The model under review builds one solid part; all positions refer to its coordinate system, in mm. A direction names the side the tool comes from. Give positions to 0.01 mm unless a question says otherwise; leave off trailing zeros. Loops run counter-clockwise (first coordinate to the right, second up) from the corner with the lowest first, then second, coordinate; pieces in that order, holes last. Notation, with made-up numbers: M 89,75.5 L 130,75.5 A35 cw 130,111.5 Z; hole C 37.5,45 d1. An arc over 180 degrees is marked long. Put each result on its own line as item: value. Start each with the question number.
from build123d import *

# Parameters (mm, degrees)
BOSS_EXTRUDE1_DEPTH     = 24
SKETCH2_R               = 2.05
SKETCH2_R_2             = 4
CUT_EXTRUDE1_DEPTH      = 45
CUT_EXTRUDE2_DEPTH      = 44.9089968
CUT_EXTRUDE2_DEPTH_BACK = 44.9089968
SKETCH3_R               = 4
SKETCH3_R_2             = 2
FILLET1_R               = 2


with BuildPart() as part:
    # Sketch1 → Boss-Extrude1 (new body)
    with BuildSketch(Plane.XY):
        Polygon((0, 0), (0, 26), (0, 28), (26, 28), (26, 26), (2, 26), (2, 2), (26, 2), (26, 0), align=None)
    extrude(amount=BOSS_EXTRUDE1_DEPTH)

    # Sketch2 → Cut-Extrude1 (cut, through all)
    with BuildSketch(Plane(origin=(2, 0, 0), x_dir=(0, 0, -1), z_dir=(1, 0, 0))):
        with Locations(Location((-12, 22, 0), (0, 0, 90))):
            Circle(SKETCH2_R)
        with Locations(Location((-12, 14, 0), (0, 0, 90))):
            Circle(SKETCH2_R_2)
        with Locations(Location((-6.343145751, 19.656854249, 0), (0, 0, 90))):
            Circle(SKETCH2_R)
        with Locations(Location((-4, 14, 0), (0, 0, 90))):
            Circle(SKETCH2_R)
        with Locations(Location((-6.343145751, 8.343145751, 0), (0, 0, 90))):
            Circle(SKETCH2_R)
        with Locations(Location((-12, 6, 0), (0, 0, 90))):
            Circle(SKETCH2_R)
        with Locations(Location((-17.656854249, 8.343145751, 0), (0, 0, 90))):
            Circle(SKETCH2_R)
        with Locations(Location((-20, 14, 0), (0, 0, 90))):
            Circle(SKETCH2_R)
        with Locations(Location((-17.656854249, 19.656854249, 0), (0, 0, 90))):
            Circle(SKETCH2_R)
    extrude(amount=-CUT_EXTRUDE1_DEPTH, mode=Mode.SUBTRACT)

    # Sketch3 → Cut-Extrude2 (cut, two sides: drawn at the far end of the back side and taken through both)
    with BuildSketch(Plane(origin=(0, 2, 0), x_dir=(1, 0, 0), z_dir=(0, 1, 0)).offset(-CUT_EXTRUDE2_DEPTH_BACK)):
        with Locations(Location((14, -12, 0), (0, 0, 270))):
            Circle(SKETCH3_R)
        with Locations(Location((22, -12, 0), (0, 0, 270))):
            Circle(SKETCH3_R_2)
        with Locations(Location((19.656854249, -17.656854249, 0), (0, 0, 270))):
            Circle(SKETCH3_R_2)
        with Locations(Location((14, -20, 0), (0, 0, 270))):
            Circle(SKETCH3_R_2)
        with Locations(Location((8.343145751, -17.656854249, 0), (0, 0, 270))):
            Circle(SKETCH3_R_2)
        with Locations(Location((6, -12, 0), (0, 0, 270))):
            Circle(SKETCH3_R_2)
        with Locations(Location((8.343145751, -6.343145751, 0), (0, 0, 270))):
            Circle(SKETCH3_R_2)
        with Locations(Location((14, -4, 0), (0, 0, 270))):
            Circle(SKETCH3_R_2)
        with Locations(Location((19.656854249, -6.343145751, 0), (0, 0, 270))):
            Circle(SKETCH3_R_2)
    extrude(amount=CUT_EXTRUDE2_DEPTH + CUT_EXTRUDE2_DEPTH_BACK, mode=Mode.SUBTRACT)

    # Fillet1
    fillet1_edges = [part.edges().sort_by_distance(p)[0] for p in [
        (26, 1, 0),
        (0, 0, 12),
        (0, 28, 12),
        (26, 27, 24),
        (26, 1, 24),
        (26, 27, 0),
    ]]
    fillet(fillet1_edges, radius=FILLET1_R)


solid = part.part
(1) Draft analysis for pull direction Y (two halves, no side actions). For faces 1 (the flat face through (17, 26, 9)), 2 (the cylindrical face through (1.014, 9.445, 19.385)), 3 (the cylindrical face through (0.57, 27.4, 12.17)), 4 (the cylindrical face through (20.8, 27, 10.4)), state which applies: +Y half, -Y half, draft (parallel to the pull), parting line (faces both ways), or undercut.
(2) We need section B-B, the plane z = 15. Write out the cut boundary in (x, y), plus the area to 3 significant figures.
(3) We need section D-D, the plane x = 23. Write out the cut boundary in (y, z), plus the area to 3 significant figures.
(4) For faces 5 (the flat face through (11, 2, 9)), 6 (the cylindrical face through (17.704, 26.986, 5.91)), list the 3-axis set-ups (+Z, -Z, +X, -X, +Y, -Y) from which the entire face can be reached by the end or side of a thin tool; tool diameter is ignored.
(5) To check wall thickness, follow L1, parallel to Z at x = 14, y = 27.55; L2, parallel to Y at x = 20.75, z = 14; L3, parallel to X at y = 26.9, z = 12. State the ranges of each line that lie inside material, in increasing order. Write a range as [from, to].
(6) We need section C-C, the plane y = 22.5. Write out the cut boundary in (x, z).
(7) Insertion check: pin 1 (6.5 mm diameter, centred on y = 19.66, z = 6.34, fed in from +X). The pin has a flat end and moves straight along its axis. Give the tip position at first contact, or say it passes through.
(8) We need section A-A, the plane x = 3. Write out the cut boundary in (y, z), plus the area to 3 significant figures.
Check sheet entries:
1. face 1: undercut
1. face 2: undercut
1. face 3: +Y half
1. face 4: draft
2. outline: M 0,2 A2 ccw 2,0 L 11.35,0 L 11.35,2 L 2,2 L 2,11.35 L 0,11.35 Z; M 0,16.65 L 2,16.65 L 2,26 L 11.35,26 L 11.35,28 L 2,28 A2 ccw 0,26 Z; M 16.65,0 L 26,0 L 26,2 L 16.65,2 Z; M 16.65,26 L 26,26 L 26,28 L 16.65,28 Z
2. area: 119 mm²
3. outline: M 0,0 L 2,0 L 2,10.27 L 0,10.27 Z; M 0,13.73 L 2,13.73 L 2,24 L 0,24 Z; M 26,0 L 28,0 L 28,10.27 L 26,10.27 Z; M 26,13.73 L 28,13.73 L 28,24 L 26,24 Z
3. area: 82.1 mm²
4. face 5: +Z, -Z, +X
4. face 6: +Y, -Y
5. L1: z = [0, 2], [6, 8], [16, 18], [22, 24]
5. L2: y = [0, 2], [26, 28]
5. L3: x = [0.21, 4], [8, 10], [18, 20], [24, 26]
6. outline: M 0,0 L 2,0 L 2,10.01 L 0,10.01 Z; M 0,13.99 L 2,13.99 L 2,24 L 0,24 Z
7. pin 1: stops at x = 2
8. outline: M 0,0 L 2,0 L 2,24 L 0,24 Z; M 26,0 L 28,0 L 28,24 L 26,24 Z
8. area: 96.0 mm²
